Could you check a few things on this model? Use its own coordinates, in mm. Face numbers are marked on the shaded views. Round coordinates to 2 decimals unless told otherwise and drop trailing zeros. Loops run counter-clockwise (first coordinate to the right, second up) from the corner with the lowest first, then second, coordinate; pieces in that order, holes last. Notation, with made-up numbers: (-31, 14.25) -> (-13, 14.25) arc R21 cw to (-13, 45.25) -> close; hole circle Ø3 at (32.25, -31.5). An arc over 180 degrees is marked (long way). One line per item, written item: value.
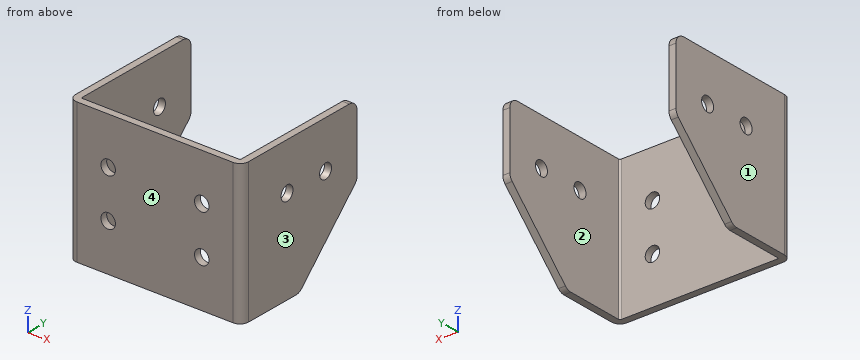
Autodesk Inventor part; units mm, degrees
ref_plane "YZ Plane" through (0, 0, 0) normal (1, 0, 0) x (0, 1, 0)
ref_plane "XZ Plane" through (0, 0, 0) normal (0, 1, 0) x (-1, 0, 0)
ref_plane "XY Plane" through (0, 0, 0) normal (0, 0, 1) x (1, 0, 0)
sketch "Sketch1" plane through (0, 0, 0) normal (0, 1, 0) x (-1, 0, 0)
  line L0 (18.5, 15) -> (-18.5, 15)
  line L1 (-18.5, 15) -> (-18.5, -15)
  line L2 (-18.5, -15) -> (18.5, -15)
  line L3 (18.5, -15) -> (18.5, 15)
  line L4 (18.5, 15) -> (-18.5, -15) construction
  line L5 (-18.5, 15) -> (18.5, -15) construction
  circle A0 centre (10, 5) radius 1.55
  circle A1 centre (10, -5) radius 1.55
  circle A2 centre (-10, 5) radius 1.55
  circle A3 centre (-10, -5) radius 1.55
  point P0 (0, 0)
  dimension "d0" = 37
  dimension "d1" = 30
  dimension "d2" = 3.1
  dimension "d3" = 3.1
  dimension "d4" = 3.1
  dimension "d5" = 3.1
  dimension "d6" = 20
  dimension "d7" = 20
  dimension "d8" = 10
  dimension "d10" = 10
  dimension "d11" = 0
  dimension "d12" = 0
  dimension "d13" = 10
  dimension "d14" = 8.5
extrude "Plate1" add sketch "Sketch1" along normal blind 1.5
sketch "Sketch2" plane through (17, 0, -15) normal (1, 0, 0) x (0, 1, 0)
  line L0 (0, 30) -> (0, 0)
  line L1 (0, 0) -> (30, 0)
  line L2 (30, 0) -> (30, 30)
  line L3 (30, 30) -> (0, 30)
edge flange "Flange1" height 30 angle 90 thickness 1.5 bend radius 0.31 thickness toward (1, 0, 0) relief tear relief width 1.5 relief depth 0.75 corner gap 0.31 corner form 0 edges at (18.5, 1.5, 0) (-18.5, 1.5, 0) wall of the first edge with corners at (17, 0, 15) (17, 0, -15) (17, 30, -15) (17, 30, 15)
bend "Bend1"
corner "Corner1"
sketch "Sketch3" plane through (18.5, 30, 15) normal (1, 0, 0) x (0, 0, -1)
  circle A0 centre (10, -8.19) radius 1.55
  circle A1 centre (10, -18.19) radius 1.55
  line L0 (0, -28.19) -> (0, 0)
  line L1 (0, -28.19) -> (30, -28.19)
  point P0 (15, -30)
  dimension "d26" = 3.1
  dimension "d27" = 3.1
  dimension "d28" = 10
  dimension "d29" = 10
  dimension "d30" = 10
  dimension "d31" = 10
extrude "Cut1" cut sketch "Sketch3" against normal through all
sketch "Sketch5" plane through (18.5, 30, 15) normal (1, 0, 0) x (0, 0, -1)
  line L0 (15, 0) -> (30, -15)
  line L1 (30, -15) -> (30, 0)
  line L2 (30, 0) -> (15, 0)
  line L3 (30, 0) -> (30, -28.19)
  line L4 (0, 0) -> (30, 0)
  point P0 (15, -30)
  dimension "d36" = 15
  dimension "d37" = 15
extrude "Cut2" cut sketch "Sketch5" against normal through all
fillet "Fillet1" radius 2 6 edges at (17.75, 30, 15) (17.75, 30, 0) (17.75, 15, -15) (-17.75, 30, 15) (-17.75, 30, 0) (-17.75, 15, -15)
equation "\"d7\" = d6"
equation "\"d10\" = d8"
equation "\"d32\" = Thickness"
equation "\"d38\" = Thickness"
equation "\"d15\" = Thickness"
equation "\"d16\" = BendReliefWidth"
equation "\"d17\" = BendReliefDepth"
equation "\"d18\" = MinimumRemnant"
equation "\"d19\" = TransitionRadius"
equation "\"d22\" = BendRadius"
equation "\"d23\" = CornerReliefSize"
equation "\"d24\" = GapSize"
equation "\"d25\" = JacobiRadiusSize"
equation "\"BendReliefWidth\" = Thickness"
equation "\"BendReliefDepth\" = 0.5 * Thickness"
equation "\"CornerReliefSize\" = 4 * Thickness"
equation "\"MinimumRemnant\" = 2 * Thickness"
equation "\"TransitionRadius\" = BendRadius"
equation "\"JacobiRadiusSize\" = BendRadius"
equation "\"GapSize\" = Thickness"
properties part number "Head1" material "Aluminum 6061-AHC"
(1) If we section it at C-C, the plane z = -5: Please give me the cut outline in (x, y), then the cut area to 3 significant figures.
Recorded:
outline: (-18.5, 1.81) arc R1.81 ccw to (-16.69, 0) -> (-11.55, 0) -> (-11.55, 1.5) -> (-16.69, 1.5) arc R0.31 cw to (-17, 1.81) -> (-17, 25) -> (-18.5, 25) -> close; (-8.45, 0) -> (8.45, 0) -> (8.45, 1.5) -> (-8.45, 1.5) -> close; (11.55, 0) -> (16.69, 0) arc R1.81 ccw to (18.5, 1.81) -> (18.5, 25) -> (17, 25) -> (17, 1.81) arc R0.31 cw to (16.69, 1.5) -> (11.55, 1.5) -> close
area: 115 mm²
(2) I'm going to push a flat-ended pin straight in: pin 1 Ø3.5 at (x, z) = (-10, 5) entering from +Y. Where does the tip first touch, or does it pass through?
Recorded:
pin 1: y = 1.5
(3) If we section it at A-A, the plane y = 21.81: Please give me the cut outline in (x, z), then the cut area to 3 significant figures.
Recorded:
outline: (-18.5, -8.19) -> (-17, -8.19) -> (-17, 3.45) -> (-18.5, 3.45) -> close; (-18.5, 6.55) -> (-17, 6.55) -> (-17, 15) -> (-18.5, 15) -> close; (17, -8.19) -> (18.5, -8.19) -> (18.5, 3.45) -> (17, 3.45) -> close; (17, 6.55) -> (18.5, 6.55) -> (18.5, 15) -> (17, 15) -> close
area: 60.3 mm²
(4) If I drill on L1, parallel to Z at x = 10, y = 0.85; L2, parallel to X at y = 23.5, z = 8.75; L3, parallel to Y at x = -4, z = 10.5, over which ranges is the centre line in solid material (lowest first)?
Recorded:
L1: -15 to -6.55, -3.45 to 3.45, 6.55 to 15
L2: -18.5 to -17, 17 to 18.5
L3: 0 to 1.5
(5) If we section it at B-B, the plane x = -10: Please give me the cut outline in (y, z), then the cut area to 3 significant figures.
Recorded:
outline: (0, -15) -> (1.5, -15) -> (1.5, -6.55) -> (0, -6.55) -> close; (0, -3.45) -> (1.5, -3.45) -> (1.5, 3.45) -> (0, 3.45) -> close; (0, 6.55) -> (1.5, 6.55) -> (1.5, 15) -> (0, 15) -> close
area: 35.7 mm²
(6) If we section it at D-D, the plane y = 11.81: Please give me the cut outline in (x, z), then the cut area to 3 significant figures.
Recorded:
outline: (-18.5, -15) -> (-17, -15) -> (-17, 3.45) -> (-18.5, 3.45) -> close; (-18.5, 6.55) -> (-17, 6.55) -> (-17, 15) -> (-18.5, 15) -> close; (17, -15) -> (18.5, -15) -> (18.5, 3.45) -> (17, 3.45) -> close; (17, 6.55) -> (18.5, 6.55) -> (18.5, 15) -> (17, 15) -> close
area: 80.7 mm²
(7) Thinking about a two-plate mould opening in X: for the marked faces 1, 2, 3 and 4, which applies, released by +X, released by -X, zero draft, split by the parting line, or undercut?
Recorded:
face 1: released by -X
face 2: undercut
face 3: released by +X
face 4: zero draft
